The model under review builds one solid part; all positions refer to its coordinate system, in mm. Coordinates: 2 decimals unless noted, no trailing zeros. Loops run counter-clockwise (first coordinate to the right, second up) from the corner with the lowest first, then second, coordinate; pieces in that order, holes last. Notation, with made-up numbers: M 26,-34 L 85,-34 A18 ccw 85,-26 Z; hole C -35.75,13 d3. An arc over 180 degrees is marked long. Return JSON: item names as keys, results as strings.
```python
from build123d import *

# Parameters (mm, degrees)
F1_DEPTH = 10


with BuildPart() as f1:
    # F0 (on Front) → F1 (new body)
    with BuildSketch(Plane.XZ):
        with BuildLine():
            Line((-55.9, -37.5), (-44.648994, -37.5))
            ThreePointArc((-44.648994, -37.5), (-42.622223, -36.711832), (-41.660409, -34.761467))
            Line((-41.660409, -34.761467), (-39.316447, -7.969854))
            ThreePointArc((-39.316447, -7.969854), (-32.58351, -0.763255), (-23.971151, -5.568959))
            ThreePointArc((-23.971151, -5.568959), (-14.391092, -17.154017), (0, -21.5))
            ThreePointArc((0, -21.5), (14.391092, -17.154017), (23.971151, -5.568959))
            ThreePointArc((23.971151, -5.568959), (32.58351, -0.763255), (39.316447, -7.969854))
            Line((39.316447, -7.969854), (41.660409, -34.761467))
            ThreePointArc((41.660409, -34.761467), (42.622223, -36.711832), (44.648994, -37.5))
            Line((44.648994, -37.5), (55.9, -37.5))
            Line((55.9, -37.5), (55.9, 4.5))
            Line((55.9, 4.5), (94.1, 4.5))
            Line((94.1, 4.5), (94.1, -37.5))
            Line((94.1, -37.5), (107.001687, -37.5))
            ThreePointArc((107.001687, -37.5), (109.028457, -36.711832), (109.990271, -34.761467))
            Line((109.990271, -34.761467), (115, 22.5))
            ThreePointArc((115, 22.5), (110.606602, 33.106602), (100, 37.5))
            Line((100, 37.5), (0, 37.5))
            Line((0, 37.5), (-100, 37.5))
            ThreePointArc((-100, 37.5), (-110.606602, 33.106602), (-115, 22.5))
            Line((-115, 22.5), (-109.990271, -34.761467))
            ThreePointArc((-109.990271, -34.761467), (-109.028457, -36.711832), (-107.001687, -37.5))
            Line((-107.001687, -37.5), (-94.1, -37.5))
            Line((-94.1, -37.5), (-94.1, 4.5))
            Line((-94.1, 4.5), (-55.9, 4.5))
            Line((-55.9, 4.5), (-55.9, -37.5))
        make_face()
        with BuildLine():
            ThreePointArc((0, -2), (-6.5, 4.5), (0, 11))
            ThreePointArc((0, 11), (6.5, 4.5), (0, -2))
        make_face(mode=Mode.SUBTRACT)
    extrude(amount=F1_DEPTH)


solid = f1.part
```
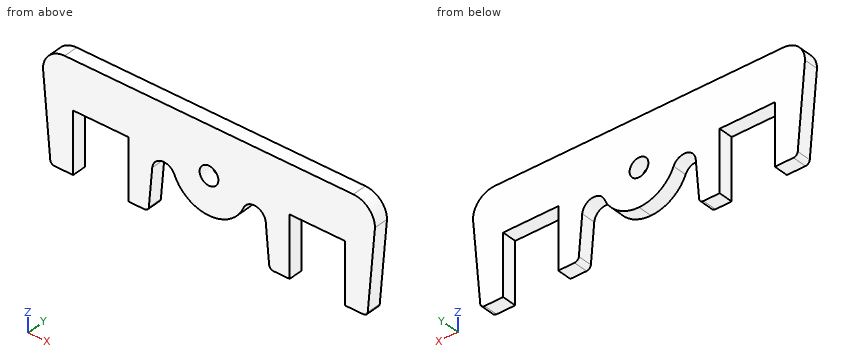
1. Add section C-C on z = -25. Give the boundary of the cut face in (x, y).
Check values:
{"outline": "M -110.84,-10 L -94.1,-10 L -94.1,0 L -110.84,0 Z; M -55.9,-10 L -40.81,-10 L -40.81,0 L -55.9,0 Z; M 40.81,-10 L 55.9,-10 L 55.9,0 L 40.81,0 Z; M 94.1,-10 L 110.84,-10 L 110.84,0 L 94.1,0 Z"}
2. Insertion check: pin 1 Ø1 at (x, y) = (67.5, -7) entering from -Z; pin 2 Ø3 at (y, z) = (-3, -22.5) entering from -X; pin 3 Ø3 at (y, z) = (-6.5, -23.5) entering from +X. Each pin has a flat end and moves straight along its axis. Give the tip position at first contact, or say it passes through.
Check values:
{"pin 1": "z = 4.5", "pin 2": "x = -111.19", "pin 3": "x = 111.11"}
3. Add section D-D on x = -78. Give the boundary of the cut face in (y, z), plus the area to 3 significant figures.
Check values:
{"outline": "M -10,4.5 L 0,4.5 L 0,37.5 L -10,37.5 Z", "area": "330 mm²"}
4. To check wall thickness, follow line 1 (X direction, y = -0.5, z = -7.5); line 2 (X direction, y = -2.75, z = 2.5); line 3 (X direction, y = -6.75, z = -13.5). State the ranges of each line that lie inside material, in increasing order.
Check values:
{"line 1": "-112.38 to -94.1, -55.9 to -39.26, -23.07 to 23.07, 39.26 to 55.9, 94.1 to 112.38", "line 2": "-113.25 to -94.1, -55.9 to -6.18, 6.18 to 55.9, 94.1 to 113.25", "line 3": "-111.85 to -94.1, -55.9 to -39.8, -18.76 to 18.76, 39.8 to 55.9, 94.1 to 111.85"}
5. Add section A-A on y = -5.75. Give the boundary of the cut face in (x, z).
Check values:
{"outline": "M -115,22.5 L -109.99,-34.76 A3 ccw -107,-37.5 L -94.1,-37.5 L -94.1,4.5 L -55.9,4.5 L -55.9,-37.5 L -44.65,-37.5 A3 ccw -41.66,-34.76 L -39.32,-7.97 A8 cw -23.97,-5.57 A26 ccw 0,-21.5 A26 ccw 23.97,-5.57 A8 cw 39.32,-7.97 L 41.66,-34.76 A3 ccw 44.65,-37.5 L 55.9,-37.5 L 55.9,4.5 L 94.1,4.5 L 94.1,-37.5 L 107,-37.5 A3 ccw 109.99,-34.76 L 115,22.5 A15 ccw 100,37.5 L -100,37.5 A15 ccw Z; hole C 0,4.5 d13"}
6. Add section B-B on z = -15. Give the boundary of the cut face in (x, y), plus the area to 3 significant figures.
Check values:
{"outline": "M -111.72,-10 L -94.1,-10 L -94.1,0 L -111.72,0 Z; M -55.9,-10 L -39.93,-10 L -39.93,0 L -55.9,0 Z; M -17.2,-10 L 17.2,-10 L 17.2,0 L -17.2,0 Z; M 39.93,-10 L 55.9,-10 L 55.9,0 L 39.93,0 Z; M 94.1,-10 L 111.72,-10 L 111.72,0 L 94.1,0 Z", "area": "1,020 mm²"}
